Read the model definition and answer for the solid it produces. Units are mm, in the model's axes. A direction names the side the tool comes from. Coordinates: 2 decimals unless noted, no trailing zeros. Write each loop counter-clockwise with the first axis right and the second up, starting at its lowest first coordinate (ties: lowest second). Pieces come first, ordered by that corner, then holes.
Item 1: Each of these flat-tipped pins is pushed along its axis until it touches: P1, Ø6, axis at y = -8.5, z = 3.5, coming from the -X side; P2, Ø2, axis at x = 5, y = -1.5, coming from the +Z side; P3, Ø6, axis at y = -1.5, z = -6.5, coming from the -X side. Where does it stop, or does it pass through?
Item 2: A tool of negligible diameter and unlimited length cuts with its end or side. For faces 1 (the face through (0, 0, 0)), 2 (the face through (1.352, -7.958, 4.292)), from which of +Z, -Z, +X, -X, +Y, -Y can it reach the whole face along a straight path? Write none if from no direction.
Item 3: Section A-A (z = 0) is taken. Give the vertices of the cut face in (x, y), then the cut area to 3 significant figures.
Item 4: Section B-B (x = 0) is taken. Give the vertices of the cut face in (y, z), then the cut area to 3 significant figures.
Item 5: Section D-D (y = -9) is taken. Give the vertices of the cut face in (x, z).
Item 6: Straight lines are drawn through the part: probe 1 along X at (y, z) = (-4, -6); probe 2 along Y at (x, z) = (5, -3.25); probe 3 along X at (y, z) = (-4, 3.75). For each, find the intervals that lie inside material, in ascending order.
Item 7: Section C-C (y = -1.25) is taken. Give the vertices of the cut face in (x, z), then the cut area to 3 significant figures.
from build123d import *

# Parameters (mm, degrees)
SKETCH_2_R      = 10
EXTRUDE_1_DEPTH = 5
SKETCH_3_R      = 4.5
EXTRUDE_2_DEPTH = 11
CHAMFER_1_SIZE  = 2


with BuildPart() as part:
    # 草圖2 → 填料-伸長1 (new body)
    with BuildSketch(Plane(origin=(0, 0, 0), x_dir=(1, 0, 0), z_dir=(0, 1, 0))):
        with Locations(Location((0, 0, 0), (0, 0, 270))):
            Circle(SKETCH_2_R)
    extrude(amount=-EXTRUDE_1_DEPTH)

    # 草圖3 → 填料-伸長2 (add)
    with BuildSketch(Plane(origin=(0, 0, 0), x_dir=(1, 0, 0), z_dir=(0, 1, 0))):
        with Locations(Location((0, 0, 0), (0, 0, 270))):
            Circle(SKETCH_3_R)
    extrude(amount=-EXTRUDE_2_DEPTH)

    # 導角1
    chamfer_1_edges = [part.edges().sort_by_distance(p)[0] for p in [
        (0, 0, -10),
    ]]
    chamfer(chamfer_1_edges, length=CHAMFER_1_SIZE)


solid = part.part
Established:
1. P1: stops at x = -4.47
1. P2: stops at z = 9.11
1. P3: stops at x = -9.35
2. face 1: +Z, -Z, +X, -X, +Y
2. face 2: -Y
3. outline: (-10, -5) - (-4.5, -5) - (-4.5, -11) - (4.5, -11) - (4.5, -5) - (10, -5) - (10, -2) - (8, 0) - (-8, 0) - (-10, -2) - close
3. area: 150 mm2
4. outline: (-11, -4.5) - (-5, -4.5) - (-5, -10) - (-2, -10) - (0, -8) - (0, 8) - (-2, 10) - (-5, 10) - (-5, 4.5) - (-11, 4.5) - close
4. area: 150 mm2
5. outline: circle Ø9 at (0, 0)
6. probe 1: x = -8 to 8
6. probe 2: y = -5 to 0
6. probe 3: x = -9.27 to 9.27
7. outline: circle Ø18.5 at (0, 0)
7. area: 269 mm2
